Check sheet for the modelled part. Datum: model origin and axes. Units: mm. A direction names the side the tool comes from. Give positions to 0.01 mm unless a question says otherwise; leave off trailing zeros. Loops run counter-clockwise (first coordinate to the right, second up) from the corner with the lowest first, then second, coordinate; pieces in that order, holes last. Notation, with made-up numbers: (-26, -24.5) -> (22, -24.5) arc R16 ccw to (22, -0.5) -> close; hole circle Ø8 at (68, 9.5). An arc over 180 degrees is marked (long way). Write each question's results on one line, items separated by ' | '. Start each with the question number.
1. Cross-section at A-A on z = -9.5. Record the boundary of the cut face in (x, y).
2. Mould release check, pull along X, two halves, no side actions. Record for faces 1 (the face through (-5, 35, -18.62)), 2 (the face through (-6, 3, -33.197)), 3 (the face through (41.044, 1, -27)), 4 (the face through (-5, -27, -18.62)): +X half, -X half, draft (parallel to the pull), parting line (faces both ways), or undercut.
3. Tool access check on faces 5 (the face through (-23.932, 2.812, -5.303)), 6 (the face through (-6, -44.881, -20)), 7 (the face through (-22.219, 6, -9)). Record the directions out of +Z, -Z, +X, -X, +Y, -Y that give a thin tool (end or side, any length) a straight path to the whole face; none if there is none.
4. Material ranges on L1, parallel to Y at x = 26, z = -10; L2, parallel to Z at x = 2.5, y = -3; L3, parallel to X at y = -22, z = -1.5, recorded low to high. Write a range as from..to.
5. Cross-section at B-B on y = -36. Record the boundary of the cut face in (x, z).
6. Gauge pin test, flat ends, axial feed: pin 1 Ø3 at (y, z) = (-3, -9) entering from +X; pin 2 Ø5 at (x, y) = (-6, 29.5) entering from +Z; pin 3 Ø11.5 at (x, y) = (-3.5, -26.5) entering from +Z; pin 4 Ø4 at (y, z) = (-20, -12.5) entering from +X. Record the tip position at first contact, or that the pin passes through.
7. Cross-section at C-C on x = -7. Record the boundary of the cut face in (y, z), and give its area (3 significant figures).
8. Cross-section at D-D on y = 5. Record the boundary of the cut face in (x, z).
from build123d import *

# Parameters (mm, degrees)
F0_W     = 93.5896597803
F0_H     = 94.0682813525
F1_DEPTH = 33.197
F2_W     = 63.2629562169
F2_H     = 40.9446330741
F3_DEPTH = 18.96077
F4_F1_R  = 7.62
F4_F2_R  = 7.62
F6_DEPTH = 123.1075


with BuildPart() as f1:
    # F0 (on Top) → F1 (new body)
    with BuildSketch(Plane.XY):
        with Locations((-5.7506207377, 2.1532103419)):
            Rectangle(F0_W, F0_H)
    extrude(amount=-F1_DEPTH)

    # F2 (on face) → F3 (cut)
    with BuildSketch(Plane.XY):
        with Locations((9.412731044, 6.3009518199)):
            Rectangle(F2_W, F2_H)
    extrude(amount=-F3_DEPTH, mode=Mode.SUBTRACT)

    # F4: fillet of radius 7.62 on 5 edges, made by hand

    # F4_f1
    f4_f1_edges = [f1.edges().sort_by_distance(p)[0] for p in [
        (9.412731044, -14.1713647172, -18.96077),
        (9.412731044, 26.7732683569, -18.96077),
        (-22.2187470645, 6.3009518199, -18.96077),
    ]]
    fillet(f4_f1_edges, radius=F4_F1_R)

    # F4_f2
    f4_f2_edges = [f1.edges().sort_by_distance(p)[0] for p in [
        (41.0442091525, 6.3009518199, -18.96077),
        (-22.2187470645, 6.3009518199, 0),
        (41.0442091525, -11.9395183898, -16.7289236726),
        (41.0442091525, 24.5414220296, -16.7289236726),
    ]]
    fillet(f4_f2_edges, radius=F4_F2_R)

    # F5 (on face) → F6 (cut)
    with BuildSketch(Plane(origin=(0, 49.1873510182, 0), x_dir=(-1, 0, 0), z_dir=(0, 1, 0))):
        Polygon((29.3431449682, 0), (-21.4069634676, 0), (0, -18.6201948673), (10.3417439386, -18.6201948673), align=None)
    extrude(amount=-F6_DEPTH, mode=Mode.SUBTRACT)


solid = f1.part
Geometry says:
1) outline: (-52.55, -44.88) -> (-19.65, -44.88) -> (-19.65, -14.17) -> (-22.22, -14.17) -> (-22.22, 26.77) -> (-19.65, 26.77) -> (-19.65, 49.19) -> (-52.55, 49.19) -> close; (10.49, -44.88) -> (41.04, -44.88) -> (41.04, -21.79) arc R7.62 ccw to (33.42, -14.17) -> (10.49, -14.17) -> close; (10.49, 26.77) -> (33.42, 26.77) arc R7.62 ccw to (41.04, 34.39) -> (41.04, 49.19) -> (10.49, 49.19) -> close
2) face 1: undercut | face 2: draft | face 3: +X half | face 4: undercut
3) face 5: +Z, +Y, -Y | face 6: +Z, -Z, +X, -X, -Y | face 7: +Z, +X
4) L1: -44.88..-14.17, 26.77..49.19 | L2: -33.2..-18.96 | L3: -52.55..-27.81, 19.68..41.04
5) outline: (-52.55, -33.2) -> (41.04, -33.2) -> (41.04, 0) -> (21.41, 0) -> (0, -18.62) -> (-10.34, -18.62) -> (-29.34, 0) -> (-52.55, 0) -> close
6) pin 1: x = -22.22 | pin 2: z = -18.62 | pin 3: z = -16.66 | pin 4: x = 41.04
7) outline: (-44.88, -33.2) -> (49.19, -33.2) -> (49.19, -18.62) -> (21.41, -18.62) arc R7.62 cw to (19.15, -18.96) -> (-6.55, -18.96) arc R7.62 cw to (-8.8, -18.62) -> (-44.88, -18.62) -> close | area: 1,360 mm^2
8) outline: (-52.55, -33.2) -> (41.04, -33.2) -> (41.04, -26.58) arc R7.62 ccw to (33.42, -18.96) -> (-14.6, -18.96) arc R7.62 cw to (-22.22, -11.34) -> (-22.22, -7.62) arc R7.62 ccw to (-22.25, -6.95) -> (-29.33, -0.02) arc R7.62 ccw to (-29.84, 0) -> (-52.55, 0) -> close
